For this review, take the finished solid that the model builds, in its own axes (mm). Round coordinates to 2 decimals unless told otherwise and drop trailing zeros. Order: outer loops, then holes, each group sorted by start corner. A loop starts at its lowest first (then second) coordinate and runs counter-clockwise, first axis right, second up. Notation, with made-up numbers: (23, -26) -> (81, -26) arc R12 cw to (81, -21) -> close; hole circle Ø1 at (74.25, 78.25). An arc over 180 degrees is marked (long way). Use a Markdown table: item, result. Add a question column.
1) Consider section C-C (z = -11.5). State the section outline as (x, y) points, plus the area to 3 significant figures.
2) Consider section A-A (y = 0). State the section outline as (x, z) points.
3) Clearance check with flat-ended pins moving along their axes: P1, Ø1.5, axis at x = -2.8, z = -32.5, coming from the -Y side; P2, Ø0.7, axis at x = -1.5, y = 4, coming from the +Z side; P3, Ø1.4, axis at x = -3.5, z = 42.5, coming from the +Y side; P4, Ø1.3, axis at y = 0.5, z = -15, coming from the +X side. State where each tip first meets the part, or that it passes through.
4) Wall thickness on line 1 along X through (y, z) = (0.75, 32.5); line 2 along Z through (x, y) = (-3.25, -4.25); line 3 along Y through (x, z) = (-2.45, 3.5): over which ranges is each line inside the solid? List them lowest first. Write a range as [from, to].
5) Consider section B-B (z = 32.5). State the section outline as (x, y) points.
```python
from build123d import *

# Parameters (mm, degrees)
EXTRUDE_1_DEPTH     = 5
CUT_EXTRUDE_1_DEPTH = 2.8
CUT_EXTRUDE_2_DEPTH = 49.765382189
SKETCH_6_W          = 5
SKETCH_6_H          = 21.25
EXTRUDE_2_DEPTH     = 2
SKETCH_5_R          = 0.85
CUT_EXTRUDE_4_DEPTH = 50.528400943
CHAMFER_1_SIZE      = 0.4


with BuildPart() as part:
    # 草图1 → 凸台-拉伸1 (new body)
    with BuildSketch(Plane(origin=(0, 0, 0), x_dir=(0, 0, -1), z_dir=(1, 0, 0))):
        Polygon((-27, 5), (27, 5), (27, 3), (48.25, 3), (48.25, -3), (27, -3), (27, -5), (-27, -5), (-27, -3), (-48.25, -3), (-48.25, 3), (-27, 3), align=None)
    extrude(amount=-EXTRUDE_1_DEPTH)

    # 草图1<3> → 切除-拉伸1 (cut)
    with BuildSketch(Plane(origin=(0, 0, 0), x_dir=(0, 0, -1), z_dir=(1, 0, 0))):
        with BuildLine():
            Line((-15.5, 2.25), (15.5, 2.25))
            ThreePointArc((15.5, 2.25), (17.75, 0), (15.5, -2.25))
            Line((15.5, -2.25), (-15.5, -2.25))
            ThreePointArc((-15.5, -2.25), (-17.75, 0), (-15.5, 2.25))
        make_face()
    extrude(amount=-CUT_EXTRUDE_1_DEPTH, mode=Mode.SUBTRACT)

    # 草图1<4> → 切除-拉伸2 (cut, through all)
    with BuildSketch(Plane(origin=(0, 0, 0), x_dir=(0, 0, -1), z_dir=(1, 0, 0))):
        with BuildLine():
            Line((-12.3, 2.25), (12.3, 2.25))
            ThreePointArc((12.3, 2.25), (14.55, 0), (12.3, -2.25))
            Line((12.3, -2.25), (-12.3, -2.25))
            ThreePointArc((-12.3, -2.25), (-14.55, 0), (-12.3, 2.25))
        make_face()
    extrude(amount=-CUT_EXTRUDE_2_DEPTH, mode=Mode.SUBTRACT)

    # 草图6 → 凸台-拉伸2 (add)
    with BuildSketch(Plane.XZ.offset(3)):
        with Locations((-2.5, -37.625)):
            Rectangle(SKETCH_6_W, SKETCH_6_H)
        with Locations((-2.5, 37.625)):
            Rectangle(SKETCH_6_W, SKETCH_6_H)
    extrude(amount=EXTRUDE_2_DEPTH)

    # 草图5 → 切除-拉伸4 (cut, through all)
    with BuildSketch(Plane.XZ.offset(5)):
        with Locations(Location((-2.8, 32.5, 0), (0, 0, 270))):
            Circle(SKETCH_5_R)
        with Locations(Location((-2.8, -32.5, 0), (0, 0, 270))):
            Circle(SKETCH_5_R)
    extrude(amount=-CUT_EXTRUDE_4_DEPTH, mode=Mode.SUBTRACT)

    # 倒角1
    chamfer_1_edges = [part.edges().sort_by_distance(p)[0] for p in [
        (0, 3, 37.625),
        (0, -5, 0),
        (0, 3, -37.625),
    ]]
    chamfer(chamfer_1_edges, length=CHAMFER_1_SIZE)


solid = part.part
```
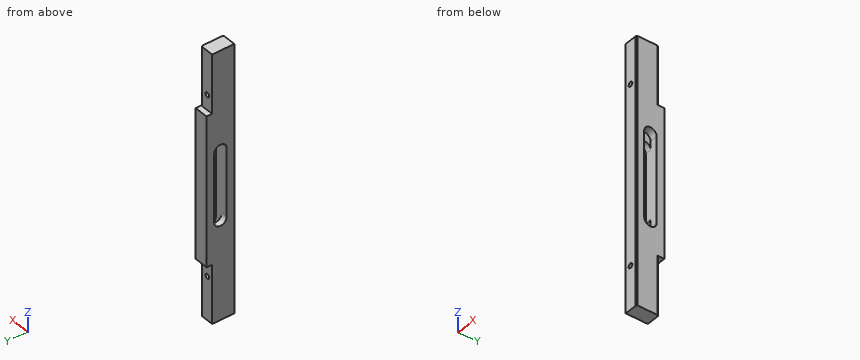
Results list:
| question | item | result |
|---|---|---|
| 1 | outline | (-5, -5) -> (-0.4, -5) -> (0, -4.6) -> (0, -2.25) -> (-5, -2.25) -> close; (-5, 2.25) -> (0, 2.25) -> (0, 5) -> (-5, 5) -> close |
| 1 | area | 27.4 mm2 |
| 2 | outline | (-5, -48.25) -> (0, -48.25) -> (0, -17.75) -> (-2.8, -17.75) -> (-2.8, -14.55) -> (-5, -14.55) -> close; (-5, 14.55) -> (-2.8, 14.55) -> (-2.8, 17.75) -> (0, 17.75) -> (0, 48.25) -> (-5, 48.25) -> close; hole circle Ø1.7 at (-2.8, -32.5); hole circle Ø1.7 at (-2.8, 32.5) |
| 3 | P1 | through |
| 3 | P2 | z = 27 |
| 3 | P3 | y = 3 |
| 3 | P4 | x = -2.8 |
| 4 | line 1 | [-5, -3.65], [-1.95, 0] |
| 4 | line 2 | [-48.25, -33.22], [-31.78, 31.78], [33.22, 48.25] |
| 4 | line 3 | [-5, -2.25], [2.25, 5] |
| 5 | outline | (-5, -5) -> (-3.65, -5) -> (-3.65, 3) -> (-5, 3) -> close; (-1.95, -5) -> (-0.4, -5) -> (0, -4.6) -> (0, 2.6) -> (-0.4, 3) -> (-1.95, 3) -> close |
